CAD build for the part. Positions are in the model's coordinates, mm. A direction names the side the tool comes from. Give positions to 0.01 mm unless a question says otherwise; leave off trailing zeros. One line per question, with ' | ' between items.
Autodesk Inventor part; units mm, degrees
ref_plane "C1_XY" through (0, 0, 0) normal (0, 0, 1) x (1, 0, 0)
ref_plane "C1_YZ" through (0, 0, 0) normal (1, 0, 0) x (0, 1, 0)
ref_plane "C1_ZX" through (0, 0, 0) normal (0, 1, 0) x (0, 0, 1)
sketch "Sketch_75" plane through (0, 0, 0) normal (0, 0, 1) x (1, 0, 0)
  line L0 (-10, -3) -> (-10, -9)
  arc A0 (-10, -9) -> (-9, -10) centre (-9, -9) ccw
  line L1 (-9, -10) -> (-3, -10)
  line L2 (-3, -10) -> (-3, -8)
  line L3 (-3, -8) -> (-6, -8)
  line L4 (-6, -8) -> (-6, -7.0607)
  line L5 (-6, -7.0607) -> (-2.9393, -4)
  line L6 (-2.9393, -4) -> (-0.6536, -4)
  arc A1 (-0.6536, -4) -> (-0.4036, -3.933) centre (-0.6536, -3.5) ccw
  line L7 (-0.4036, -3.933) -> (0, -3.7)
  line L8 (0, -3.7) -> (0.4036, -3.933)
  arc A2 (0.4036, -3.933) -> (0.9036, -3.933) centre (0.6536, -3.5) ccw
  line L9 (0.9036, -3.933) -> (1.2189, -3.751)
  line L10 (1.2189, -3.751) -> (2.5, -4)
  line L11 (2.5, -4) -> (2.9393, -4)
  line L12 (2.9393, -4) -> (6, -7.0607)
  line L13 (6, -7.0607) -> (6, -8)
  line L14 (6, -8) -> (3, -8)
  line L15 (3, -8) -> (3, -10)
  line L16 (3, -10) -> (9, -10)
  arc A3 (9, -10) -> (10, -9) centre (9, -9) ccw
  line L17 (10, -9) -> (10, -3)
  line L18 (10, -3) -> (8, -3)
  line L19 (8, -3) -> (8, -6)
  line L20 (8, -6) -> (7.0607, -6)
  line L21 (7.0607, -6) -> (4, -2.9393)
  line L22 (4, -2.9393) -> (4, -0.6536)
  arc A4 (4, -0.6536) -> (3.933, -0.4036) centre (3.5, -0.6536) ccw
  line L23 (3.933, -0.4036) -> (3.7, 0)
  line L24 (3.7, 0) -> (3.933, 0.4036)
  arc A5 (3.933, 0.4036) -> (3.933, 0.9036) centre (3.5, 0.6536) ccw
  line L25 (3.933, 0.9036) -> (3.751, 1.2189)
  line L26 (3.751, 1.2189) -> (4, 2.5)
  line L27 (4, 2.5) -> (4, 2.9393)
  line L28 (4, 2.9393) -> (7.0607, 6)
  line L29 (7.0607, 6) -> (8, 6)
  line L30 (8, 6) -> (8, 3)
  line L31 (8, 3) -> (10, 3)
  line L32 (10, 3) -> (10, 9)
  arc A6 (10, 9) -> (9, 10) centre (9, 9) ccw
  line L33 (9, 10) -> (3, 10)
  line L34 (3, 10) -> (3, 8)
  line L35 (3, 8) -> (6, 8)
  line L36 (6, 8) -> (6, 7.0607)
  line L37 (6, 7.0607) -> (2.9393, 4)
  line L38 (2.9393, 4) -> (0.6536, 4)
  arc A7 (0.6536, 4) -> (0.4036, 3.933) centre (0.6536, 3.5) ccw
  line L39 (0.4036, 3.933) -> (0, 3.7)
  line L40 (0, 3.7) -> (-0.4036, 3.933)
  arc A8 (-0.4036, 3.933) -> (-0.9036, 3.933) centre (-0.6536, 3.5) ccw
  line L41 (-0.9036, 3.933) -> (-1.2189, 3.751)
  line L42 (-1.2189, 3.751) -> (-2.5, 4)
  line L43 (-2.5, 4) -> (-2.9393, 4)
  line L44 (-2.9393, 4) -> (-6, 7.0607)
  line L45 (-6, 7.0607) -> (-6, 8)
  line L46 (-6, 8) -> (-3, 8)
  line L47 (-3, 8) -> (-3, 10)
  line L48 (-3, 10) -> (-9, 10)
  arc A9 (-9, 10) -> (-10, 9) centre (-9, 9) ccw
  line L49 (-10, 9) -> (-10, 3)
  line L50 (-10, 3) -> (-8, 3)
  line L51 (-8, 3) -> (-8, 6)
  line L52 (-8, 6) -> (-7.0607, 6)
  line L53 (-7.0607, 6) -> (-4, 2.9393)
  line L54 (-4, 2.9393) -> (-4, 0.6536)
  arc A10 (-4, 0.6536) -> (-3.933, 0.4036) centre (-3.5, 0.6536) ccw
  line L55 (-3.933, 0.4036) -> (-3.7, 0)
  line L56 (-3.7, 0) -> (-3.933, -0.4036)
  arc A11 (-3.933, -0.4036) -> (-3.933, -0.9036) centre (-3.5, -0.6536) ccw
  line L57 (-3.933, -0.9036) -> (-3.751, -1.2189)
  line L58 (-3.751, -1.2189) -> (-4, -2.5)
  line L59 (-4, -2.5) -> (-4, -2.9393)
  line L60 (-4, -2.9393) -> (-7.0607, -6)
  line L61 (-7.0607, -6) -> (-8, -6)
  line L62 (-8, -6) -> (-8, -3)
  line L63 (-8, -3) -> (-10, -3)
extrude "Extrusion1" add sketch "Sketch_75" against normal blind 100
sketch "Sketch2" plane through (0, 0, -100) normal (0, 0, -1) x (-1, 0, 0)
  point P0 (0, 0)
hole "Hole1" at (0, 0, -100) direction (0, 0, 1) diameter 4.2 depth 100
ref_plane "C1_XY" through (0, 0, 0) normal (0, 0, 1) x (1, 0, 0)
ref_plane "C1_YZ" through (0, 0, 0) normal (1, 0, 0) x (0, 1, 0)
ref_plane "C1_ZX" through (0, 0, 0) normal (0, 1, 0) x (0, 0, 1)
properties part number "NFS5-2020-100" material "アルミニウム 6061"
Item 1: Drill centre lines: line 1 along X through (y, z) = (-9, -77); line 2 along X through (y, z) = (0, -30); line 3 along X through (y, z) = (5.5, -49). Where is each one in solid material? Low to high. Write a range as [from, to].
Conclusion:
line 1: [-10, -3], [3, 10] | line 2: [-3.7, -2.1], [2.1, 3.7] | line 3: [-10, -8], [-6.56, -4.44], [4.44, 6.56], [8, 10]
Item 2: 3-axis set-ups, long thin cutter, end or side, ignore diameter. For faces 1 (the flat face through (3, -9, -49)), 2 (the flat face through (4, 8, -49)), 3 (the flat face through (-9, -3, -49)): which of +Z, -Z, +X, -X, +Y, -Y reach the whole face in a straight line?
Conclusion:
face 1: +Z, -Z, -Y | face 2: +Z, -Z | face 3: +Z, -Z, -X
Item 3: Drop a flat-ended pin along its axis: P1, Ø1.5, axis at x = 2, y = 7.5, coming from the +Z side. Give the stop position or say it passes through.
Conclusion:
P1: through
Item 4: Mould opens along Y. For faces 4 (the flat face through (-0.1, 2.4, -100)), 5 (the flat face through (6, -10, -49)), 6 (the flat face through (-5.55, 4.49, -49.3)) say: pulls with the +Y half, pulls with the -Y half, needs draft (parallel to the pull), parting line crosses it, or undercut.
Conclusion:
face 4: needs draft | face 5: pulls with the -Y half | face 6: undercut
